Geometry check sheet. Reference: the model listing, model coordinates, mm. A direction names the side the tool comes from. Round coordinates to 2 decimals unless told otherwise and drop trailing zeros. Order: outer loops, then holes, each group sorted by start corner. A loop starts at its lowest first (then second) coordinate and runs counter-clockwise, first axis right, second up.
(1) Go/stop test with flat-tipped pins: pin 1 (3 mm diameter, centred on x = 0, z = 6, fed in from +Y); pin 2 (3.5 mm diameter, centred on x = 19.55, y = 19.55, fed in from +Z); pin 3 (3 mm diameter, centred on y = 23, z = 11.5, fed in from +X). Record where each tip stops, or that it passes through.
(2) Material ranges on line 1 along X through (y, z) = (0, 9.5) (3 decimals); line 2 along Y through (x, z) = (-10, 6); line 3 along X through (y, z) = (0, 5.5) (3 decimals), recorded low to high.
(3) Sectioned sample at B-B (y = 23.5). Record the boundary of the cut face in (x, z), plus the area to 3 significant figures.
(4) Sectioned sample at A-A (z = 4.5). Give the number of separate pieces and of enclosed holes in the cut face, plus the area to 3 significant figures.
(5) Sectioned sample at C-C (x = 24). Record the boundary of the cut face in (y, z), plus the area to 3 significant figures.
(6) Set-up check for faces 4 (the face through (22.965, 24.906, 8.409)), 5 (the face through (-7.3, 0.729, 3.686)), 6 (the face through (17.526, 17.339, 2.028)), 7 (the face through (1.12, -7.3, 8.15)), 8 (the face through (0, 0, 20)): record each of +Z, -Z, +X, -X, +Y, -Y from which the full face is reachable in a straight line by a thin tool's end or side.
(7) Release check for a two-part mould opening along X. For faces 1 (the face through (8, 8, 0)), 2 (the face through (3.03, 0.95, 6.9)), 3 (the face through (5.86, -11.267, 7.395)) record: +X half, -X half, draft (parallel to the pull), parting line (faces both ways), or undercut.
from build123d import *

# Parameters (mm, degrees)
SKETCH1_R           = 12.7
BOSS_EXTRUDE1_DEPTH = 20
FILLET1_R           = 5
CUT_EXTRUDE1_REACH  = 14.7
SKETCH3_R           = 2.4257
CUT_EXTRUDE2_REACH  = 14.7
SKETCH4_R           = 2.4257
BOSS_EXTRUDE2_DEPTH = 2
SKETCH6_R           = 6.35
BOSS_EXTRUDE3_DEPTH = 13
SKETCH8_R           = 0.9525
CUT_EXTRUDE3_DEPTH  = 16.0000001


with BuildPart() as part:
    # Sketch1 → Boss-Extrude1 (new body)
    with BuildSketch(Plane.XY):
        Circle(SKETCH1_R)
    extrude(amount=BOSS_EXTRUDE1_DEPTH)

    # Sketch2 → Cut-Revolve1 (revolve, cut)
    with BuildSketch(Plane(origin=(0, 0, 0), x_dir=(1, 0, 0), z_dir=(0, 1, 0))):
        Polygon((0, 0), (0, -17.175), (3.175, -14), (3.175, 0), align=None)
    revolve(axis=Axis((0, 0, -1), (0, 0, 1)), mode=Mode.SUBTRACT)

    # Fillet1
    fillet1_edges = [part.edges().sort_by_distance(p)[0] for p in [
        (-12.7, 0, 20),
    ]]
    fillet(fillet1_edges, radius=FILLET1_R)

    # Sketch3 → Cut-Extrude1 (cut, up to next)
    with BuildSketch(Plane(origin=(0, 0, 0), x_dir=(1, 0, 0), z_dir=(0, 1, 0)), mode=Mode.PRIVATE) as cut_extrude1_sk1:
        with Locations((0, -6)):
            Circle(SKETCH3_R)
    cut_extrude1_tool1 = extrude(cut_extrude1_sk1.sketch, amount=-CUT_EXTRUDE1_REACH, mode=Mode.PRIVATE) & part.part
    add(cut_extrude1_tool1.solids().sort_by_distance((0, 0, 6))[0], mode=Mode.SUBTRACT)

    # Sketch4 → Cut-Extrude2 (cut, up to next)
    with BuildSketch(Plane(origin=(0, 0, 0), x_dir=(0, 0, -1), z_dir=(1, 0, 0)), mode=Mode.PRIVATE) as cut_extrude2_sk1:
        with Locations((-6, 0)):
            Circle(SKETCH4_R)
    cut_extrude2_tool1 = extrude(cut_extrude2_sk1.sketch, amount=-CUT_EXTRUDE2_REACH, mode=Mode.PRIVATE) & part.part
    add(cut_extrude2_tool1.solids().sort_by_distance((0, 0, 6))[0], mode=Mode.SUBTRACT)

    # Sketch5 → Boss-Extrude2 (add)
    with BuildSketch(Plane.XY):
        with BuildLine():
            Line((13.789783932, 26.915271857), (-7.826077627, 10.002125223))
            ThreePointArc((-7.826077627, 10.002125223), (8.980256121, 8.980256121), (10.002125223, -7.826077627))
            Line((10.002125223, -7.826077627), (26.915271857, 13.789783932))
            ThreePointArc((26.915271857, 13.789783932), (26.162950904, 26.162950904), (13.789783932, 26.915271857))
        make_face()
    extrude(amount=BOSS_EXTRUDE2_DEPTH)

    # Sketch6 → Boss-Extrude3 (add)
    with BuildSketch(Plane.XY.offset(2)):
        with Locations((19.5515025, 19.5515025)):
            Circle(SKETCH6_R)
    extrude(amount=BOSS_EXTRUDE3_DEPTH)

    # Sketch7 → Cut-Revolve2 (revolve, cut)
    with BuildSketch(Plane(origin=(0, 0, 0), x_dir=(0, 0, 1), z_dir=(-0.707106781, 0.707106781, 0))):
        Polygon((0, 30.65), (4, 30.65), (7, 27.65), (0, 27.65), align=None)
    revolve(axis=Axis((19.5515025, 19.5515025, 15), (0, 0, -1)), mode=Mode.SUBTRACT)

    # Sketch8 → Cut-Extrude3 (cut, through all)
    with BuildSketch(Plane.XY.offset(15)):
        with Locations((19.5515025, 19.5515025)):
            Circle(SKETCH8_R)
    extrude(amount=-CUT_EXTRUDE3_DEPTH, mode=Mode.SUBTRACT)


solid = part.part
Answer below:
1. pin 1: stops at y = 12.7
1. pin 2: stops at z = 15
1. pin 3: stops at x = 25.6
2. line 1: x = -12.7 to -3.175, 3.175 to 12.7
2. line 2: y = -7.83 to -2.43, 2.43 to 7.83
2. line 3: x = 3.175 to 12.7
3. outline: (9.42, 0) - (28.03, 0) - (28.03, 2) - (24.52, 2) - (24.52, 15) - (14.58, 15) - (14.58, 2) - (9.42, 2) - close
3. area: 167 mm2
4. separate pieces: 3
4. enclosed holes: 1
4. area: 508 mm2
5. outline: (10.06, 0) - (27.78, 0) - (27.78, 2) - (24.08, 2) - (24.08, 15) - (15.02, 15) - (15.02, 2) - (10.06, 2) - close
5. area: 153 mm2
6. face 4: +Z
6. face 5: -X
6. face 6: -Z
6. face 7: -Y
6. face 8: +Z, +X, -X, +Y, -Y
7. face 1: draft
7. face 2: undercut
7. face 3: parting line
